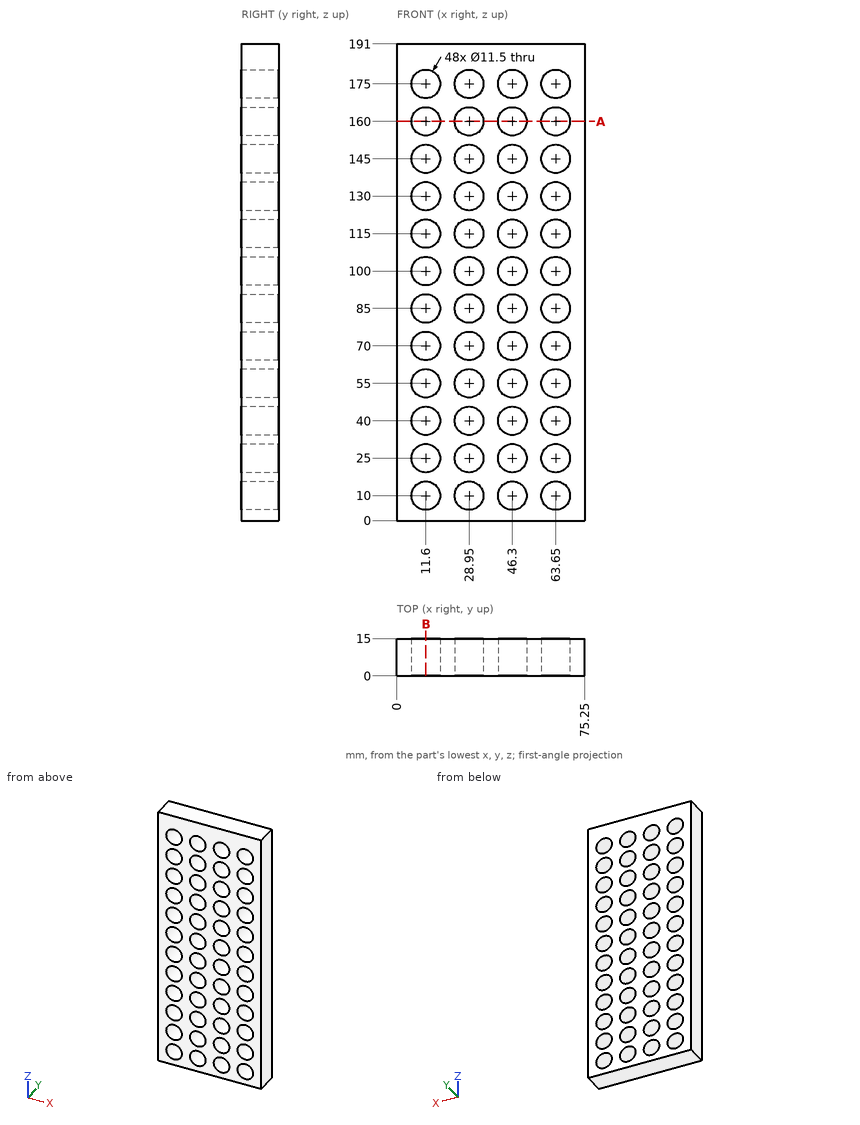
Input: dimensioned drawing with shaded views. Units: mm. Origin: part minimum x, y, z. Round coordinates to 2 decimals unless told otherwise and drop trailing zeros. Order: outer loops, then holes, each group sorted by start corner. A loop starts at its lowest first (then second) coordinate and runs counter-clockwise, first axis right, second up. Notation, with made-up numbers: (-23.75, 25) -> (29.25, 25) arc R16 cw to (29.25, 38) -> close; hole circle Ø5 at (65.25, 13.5). An arc over 180 degrees is marked (long way). Put each result on its own line as item: value. Start each with the question number.
Q1. Section A-A on z = 160. Return the cut outline in (x, y), and give its area (3 significant figures).
Q2. Line query: probe 1 along X at (y, z) = (5.5, 40); probe 2 along X at (y, z) = (7.25, 51.5). Output: solid intervals per line, ascending.
Q3. Section B-B on x = 11.6. Give the number of separate pieces and of enclosed holes in the cut face, and give its area (3 significant figures).
Ans:
1. outline: (0, 0) -> (5.85, 0) -> (5.85, 15) -> (0, 15) -> close; (17.35, 0) -> (23.2, 0) -> (23.2, 15) -> (17.35, 15) -> close; (34.7, 0) -> (40.55, 0) -> (40.55, 15) -> (34.7, 15) -> close; (52.05, 0) -> (57.9, 0) -> (57.9, 15) -> (52.05, 15) -> close; (69.4, 0) -> (75.25, 0) -> (75.25, 15) -> (69.4, 15) -> close
1. area: 439 mm2
2. probe 1: x = 0 to 5.85, 17.35 to 23.2, 34.7 to 40.55, 52.05 to 57.9, 69.4 to 75.25
2. probe 2: x = 0 to 7.04, 16.16 to 24.39, 33.51 to 41.74, 50.86 to 59.09, 68.21 to 75.25
3. separate pieces: 13
3. enclosed holes: 0
3. area: 795 mm2
